from build123d import *

# Parameters (mm, degrees)
F1_DEPTH     = 5
F3_DEPTH     = 30
F5_DEPTH     = 61
F6_W         = 41
F6_H         = 20
F6_W_2       = 15
F6_H_2       = 15
F7_DEPTH     = 4.001
F8_R         = 1.5
F9_DEPTH     = 35.001
F10_R        = 2
F11_T1_DEPTH = 8.5
F11_T3_DEPTH = 4
F11_T5_DEPTH = 59
F11_T8_ANGLE = 90


# Not quite as in the source:
# - a fillet or chamfer that OpenCascade refuses, or shapes differently, is made with other operations: its cross-section is extruded or revolved along the edge and cut away or added


with BuildPart() as f1:
    # F0 (on Top) → F1 (new body)
    with BuildSketch(Plane.XY):
        Polygon((33, 47.5), (-33, 47.5), (-33, -32.5), (14, -32.5), (14, -47.5), (33, -47.5), align=None)
    extrude(amount=F1_DEPTH)

    # F2 (on face) → F3 (join)
    with BuildSketch(Plane.XY.offset(5)):
        Polygon((-33, 42.5), (28, 42.5), (28, -47.5), (33, -47.5), (33, 47.5), (-33, 47.5), align=None)
    extrude(amount=F3_DEPTH)

    # F4 (on face) → F5 (join, through all)
    with BuildSketch(Plane(origin=(28, 0, 0), x_dir=(0, -1, 0), z_dir=(-1, 0, 0))):
        Polygon((47.5, 35), (-42.5, 35), (-42.5, 27), (-36.5, 27), (-36.5, 33), (-6.5, 33), (-6.5, 27), (8.5, 27), (8.5, 15), (19.5, 15), (19.5, 31), (37.5, 31), (37.5, 15), (47.5, 15), align=None)
    extrude(amount=F5_DEPTH)

    # F6 (on face) → F7 (cut, through all)
    with BuildSketch(Plane.XY.offset(35)):
        with Locations((-12.5, 21.5)):
            Rectangle(F6_W, F6_H)
        with Locations((12.5, -27)):
            Rectangle(F6_W_2, F6_H_2)
    extrude(amount=-F7_DEPTH, mode=Mode.SUBTRACT)

    # F8 (on face) → F9 (cut, through all)
    with BuildSketch(Plane(origin=(0, 0, 0), x_dir=(1, 0, 0), z_dir=(0, 0, -1))):
        with Locations((23.5, 42.5)):
            Circle(F8_R)
    extrude(amount=-F9_DEPTH, mode=Mode.SUBTRACT)

    # F10
    f10_edges = [f1.edges().sort_by_distance(p)[0] for p in [
        (-33, -18, 35),
        (-33, 39.5, 35),
        (-33, -19.5, 23),
        (-33, -37.5, 23),
        (-33, -8.5, 21),
        (-33, -1, 27),
        (-33, 42.5, 16),
        (-33, -32.5, 2.5),
    ]]
    fillet(f10_edges, radius=F10_R)

    # F11: fillet of radius 1 on 2 edges, made by hand

    # F11_s2 → F11_t1 (cut)
    with BuildSketch(Plane.XY.offset(24.5)):
        with BuildLine():
            ThreePointArc((-33, 37.5), (-32.7071067812, 36.7928932188), (-32, 36.5))
            Line((-32, 36.5), (-33, 36.5))
            Line((-33, 36.5), (-33, 37.5))
        make_face()
    extrude(amount=F11_T1_DEPTH, mode=Mode.SUBTRACT)

    # F11_s4 → F11_t3 (cut)
    with BuildSketch(Plane.XY.offset(29)):
        with BuildLine():
            ThreePointArc((-33, 5.5), (-32.7071067812, 6.2071067812), (-32, 6.5))
            Line((-32, 6.5), (-33, 6.5))
            Line((-33, 6.5), (-33, 5.5))
        make_face()
    extrude(amount=F11_T3_DEPTH, mode=Mode.SUBTRACT)

    # F11_s6 → F11_t5 (cut)
    with BuildSketch(Plane.YZ.offset(-31)):
        with BuildLine():
            ThreePointArc((6.5, 28), (6.2071067812, 27.2928932188), (5.5, 27))
            Line((5.5, 27), (6.5, 27))
            Line((6.5, 27), (6.5, 28))
        make_face()
    extrude(amount=F11_T5_DEPTH, mode=Mode.SUBTRACT)

    # F11_s7 → F11_t8 (revolve, cut)
    with BuildSketch(Plane.XY.offset(29)):
        with BuildLine():
            ThreePointArc((-32, 6.5), (-32.7071067812, 6.2071067812), (-33, 5.5))
            Line((-33, 5.5), (-33, 6.5))
            Line((-33, 6.5), (-32, 6.5))
        make_face()
    revolve(axis=Axis((-31, 6.5, 29), (0, -1, 0)), revolution_arc=F11_T8_ANGLE, mode=Mode.SUBTRACT)


solid = f1.part
Geometry check sheet. Reference: the model listing, model coordinates, mm. A direction names the side the tool comes from. Give positions to 0.01 mm unless a question says otherwise; leave off trailing zeros. Loops run counter-clockwise (first coordinate to the right, second up) from the corner with the lowest first, then second, coordinate; pieces in that order, holes last. Notation, with made-up numbers: (49.25, -39) -> (82.25, -39) arc R34 ccw to (82.25, -4) -> close; hole circle Ø2 at (-1, 59.5). An arc over 180 degrees is marked (long way). Answer in a Markdown table with one row per item. Add a question column.
1) Cross-section at C-C on x = 16. Record the boundary of the cut face in (y, z).
2) Cross-section at D-D on z = 20. Record the boundary of the cut face in (x, y).
3) Cross-section at B-B on y = -42.5. Record the boundary of the cut face in (x, z).
4) Material ranges on probe 1 along Y at (x, z) = (-22, 30); probe 2 along Y at (x, z) = (-8.5, 19); probe 3 along Z at (x, y) = (17, -10), recorded low to high. Write a range as from..to.
5) Gauge pin test, flat ends, axial feed: P1, Ø2.5, axis at y = -42, z = 1.5, coming from the -X side; P2, Ø0.6, axis at y = 21, z = 34.5, coming from the -X side; P3, Ø1.5, axis at x = 2.5, z = 2, coming from the -Y side. Record the tip position at first contact, or that the pin passes through.
6) Cross-section at A-A on x = 23.5. Record the boundary of the cut face in (y, z), and give its area (3 significant figures).
7) Set-up check for faces 1 (the face through (12, -34.5, 33)), 2 (the face through (-3, -1, 5)), 3 (the face through (-13, 31.5, 34)), 4 (the face through (-2, 40, 27)): record each of +Z, -Z, +X, -X, +Y, -Y from which the full face is reachable in a straight line by a thin tool's end or side.
8) Draft check along Y on faces 5 (the face through (-1, -8.5, 21)), 6 (the face through (-9, -32.5, 2)), 7 (the face through (-2, -42, 15)). Enter one of: pulls with the +Y half, pulls with the -Y half, needs draft (parallel to the pull), parting line crosses it, or undercut.
Outcome:
| question | item | result |
|---|---|---|
| 1 | outline | (-47.5, 0) -> (47.5, 0) -> (47.5, 35) -> (-19.5, 35) -> (-19.5, 15) -> (-8.5, 15) -> (-8.5, 27) -> (5.5, 27) arc R1 ccw to (6.5, 28) -> (6.5, 33) -> (36.5, 33) -> (36.5, 27) -> (42.5, 27) -> (42.5, 5) -> (-47.5, 5) -> close; (-47.5, 15) -> (-37.5, 15) -> (-37.5, 31) -> (-34.5, 31) -> (-34.5, 35) -> (-47.5, 35) -> close |
| 2 | outline | (-33, -47.5) -> (33, -47.5) -> (33, 47.5) -> (-33, 47.5) -> (-33, 44.5) arc R2 ccw to (-31, 42.5) -> (28, 42.5) -> (28, -8.5) -> (-31, -8.5) arc R2 ccw to (-33, -10.5) -> (-33, -17.5) arc R2 ccw to (-31, -19.5) -> (28, -19.5) -> (28, -37.5) -> (-31, -37.5) arc R2 ccw to (-33, -39.5) -> close; hole circle Ø3 at (23.5, -42.5) |
| 3 | outline | (-33, 15) -> (22, 15) -> (22, 35) -> (-31, 35) arc R2 ccw to (-33, 33) -> close; (14, 0) -> (22, 0) -> (22, 5) -> (14, 5) -> close; (25, 0) -> (33, 0) -> (33, 35) -> (25, 35) -> (25, 15) -> (28, 15) -> (28, 5) -> (25, 5) -> close |
| 4 | probe 1 | y = -47.5..-37.5, -19.5..6.5, 36.5..47.5 |
| 4 | probe 2 | y = -47.5..-37.5, -19.5..-8.5, 42.5..47.5 |
| 4 | probe 3 | z = 0..5, 15..35 |
| 5 | P1 | stops at x = 14 |
| 5 | P2 | stops at x = 8 |
| 5 | P3 | stops at y = -32.5 |
| 6 | outline | (-47.5, 0) -> (-44, 0) -> (-44, 5) -> (-47.5, 5) -> close; (-47.5, 15) -> (-44, 15) -> (-44, 35) -> (-47.5, 35) -> close; (-41, 0) -> (47.5, 0) -> (47.5, 35) -> (-41, 35) -> (-41, 15) -> (-37.5, 15) -> (-37.5, 31) -> (-19.5, 31) -> (-19.5, 15) -> (-8.5, 15) -> (-8.5, 27) -> (5.5, 27) arc R1 ccw to (6.5, 28) -> (6.5, 33) -> (36.5, 33) -> (36.5, 27) -> (42.5, 27) -> (42.5, 5) -> (-41, 5) -> close |
| 6 | area | 1,270 mm^2 |
| 7 | face 1 | +Z |
| 7 | face 2 | -X, -Y |
| 7 | face 3 | +Z, -X |
| 7 | face 4 | -X |
| 8 | face 5 | undercut |
| 8 | face 6 | pulls with the -Y half |
| 8 | face 7 | needs draft |
